Geometry check sheet. Reference: the model listing, model coordinates, mm. Face numbers are marked on the shaded views. A direction names the side the tool comes from. Round coordinates to 2 decimals unless told otherwise and drop trailing zeros. Loops run counter-clockwise (first coordinate to the right, second up) from the corner with the lowest first, then second, coordinate; pieces in that order, holes last.
```python
from build123d import *

# Parameters (mm, degrees)
BOSS_EXTRUDE1_DEPTH = 37
SKETCH3_W           = 1.5
SKETCH3_H           = 10
BOSS_EXTRUDE2_DEPTH = 15


with BuildPart() as part:
    # Sketch1 → Boss-Extrude1 (new body)
    with BuildSketch(Plane(origin=(0, 0, 0), x_dir=(1, 0, 0), z_dir=(0, 1, 0))):
        with BuildLine():
            ThreePointArc((-33, 0), (0, 33), (33, 0))
            Line((33, 0), (43, 0))
            ThreePointArc((43, 0), (0, 43), (-43, 0))
            Line((-43, 0), (-33, 0))
        make_face()
    extrude(amount=BOSS_EXTRUDE1_DEPTH)

    # Sketch3 → Boss-Extrude2 (add, symmetric)
    with BuildSketch(Plane(origin=(0, 18.5, 0), x_dir=(1, 0, 0), z_dir=(0, 1, 0))):
        with Locations((-40.25, -5)):
            Rectangle(SKETCH3_W, SKETCH3_H)
        Polygon((-43, -8), (-41, -10), (-41, -6), align=None)
    boss_extrude2 = extrude(amount=BOSS_EXTRUDE2_DEPTH, both=True)

    # Mirror1: Boss-Extrude2 across plane
    add(boss_extrude2.mirror(Plane(origin=(0, 0, 0), x_dir=(0, 0, 1), z_dir=(1, 0, 0))))


solid = part.part
```
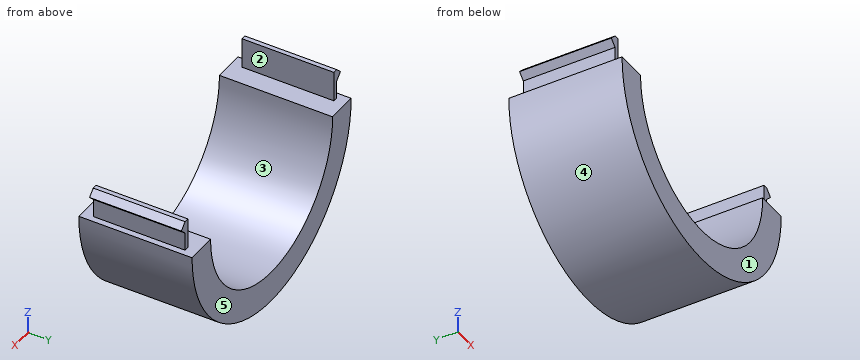
1) Sectioned sample at D-D, the plane x = 0. Record the cut outline in (y, z), then the cut area to 3 significant figures.
Report:
outline: (0, -43) - (37, -43) - (37, -33) - (0, -33) - close
area: 370 mm2
2) Scan lines: line 1 along X through (y, z) = (21, -23.5); line 2 along X through (y, z) = (20, -16); line 3 along Z through (x, y) = (-19, 2.5). Record each from-to range of solid material in increasing order.
Report:
line 1: x = -36.01 to -23.17, 23.17 to 36.01
line 2: x = -39.91 to -28.86, 28.86 to 39.91
line 3: z = -38.57 to -26.98
3) Sectioned sample at C-C, the plane z = -24. Record the cut outline in (x, y), then the cut area to 3 significant figures.
Report:
outline: (-35.68, 0) - (-22.65, 0) - (-22.65, 37) - (-35.68, 37) - close; (22.65, 0) - (35.68, 0) - (35.68, 37) - (22.65, 37) - close
area: 964 mm2
4) Access from +Z, -Z, +X, -X, +Y, -Y to the whole of each face (thin tool, end or side, straight path). Record for the marked faces 1 and 2.
Report:
face 1: +Z, -Z, +X, -X, -Y
face 2: +Z, +Y, -Y
5) Mould release check, pull along X, two halves, no side actions. Record for the marked faces 3, 4 and 5: +X half, -X half, draft (parallel to the pull), parting line (faces both ways), or undercut.
Report:
face 3: undercut
face 4: parting line
face 5: draft
6) Sectioned sample at B-B, the plane y = 11. Record the cut outline in (x, z).
Report:
outline: (-43, 0) arc R43 ccw to (43, 0) - (41, 0) - (41, 6) - (43, 8) - (41, 10) - (39.5, 10) - (39.5, 0) - (33, 0) arc R33 cw to (-33, 0) - (-39.5, 0) - (-39.5, 10) - (-41, 10) - (-43, 8) - (-41, 6) - (-41, 0) - close
7) Sectioned sample at A-A, the plane z = -16. Record the cut outline in (x, y), then the cut area to 3 significant figures.
Report:
outline: (-39.91, 0) - (-28.86, 0) - (-28.86, 37) - (-39.91, 37) - close; (28.86, 0) - (39.91, 0) - (39.91, 37) - (28.86, 37) - close
area: 818 mm2
8) Gauge pin test, flat ends, axial feed: pin 1 (1 mm diameter, centred on x = 42, z = 3.5, fed in from +Y); pin 2 (3 mm diameter, centred on x = -41.5, z = 2.5, fed in from +Y); pin 3 (3 mm diameter, centred on x = -41, z = 3.5, fed in from -Y); pin 4 (1.5 mm diameter, centred on x = 19, y = 33, fed in from -Z). Record the tip position at first contact, or that the pin passes through.
Report:
pin 1: passes through
pin 2: stops at y = 33.5
pin 3: stops at y = 3.5
pin 4: stops at z = -38.94
